Can you work these out from the model? Positions are in its coordinate system, mm. Coordinates: 2 decimals unless noted, no trailing zeros. Order: outer loops, then holes, each group sorted by start corner. A loop starts at its lowest first (then second) coordinate and runs counter-clockwise, first axis right, second up.
```python
from build123d import *

# Parameters (mm, degrees)
SKETCH1_W           = 65
SKETCH1_H           = 75
SKETCH1_R           = 2.75
SKETCH1_R_2         = 6
BOSS_EXTRUDE1_DEPTH = 5
CHAMFER1_SIZE       = 3
CUT_EXTRUDE1_REACH  = 58.789
SKETCH2_R           = 2.75
CUT_EXTRUDE2_REACH  = 58.789
SKETCH3_W           = 28
SKETCH3_H           = 20
FILLET1_R           = 40


with BuildPart() as part:
    # Sketch1 → Boss-Extrude1 (new body)
    with BuildSketch(Plane(origin=(600.828774839, 0, 0), x_dir=(0, -1, 0), z_dir=(-1, 0, 0))):
        with Locations((7.5, -2.5)):
            Rectangle(SKETCH1_W, SKETCH1_H)
        with Locations((30, -5)):
            Circle(SKETCH1_R, mode=Mode.SUBTRACT)
        with Locations(Location((-10, 25, 0), (0, 0, 180))):
            Circle(SKETCH1_R, mode=Mode.SUBTRACT)
        with Locations(Location((30, -25, 0), (0, 0, 180))):
            Circle(SKETCH1_R, mode=Mode.SUBTRACT)
        with Locations(Location((0, -10, 0), (0, 0, 180))):
            Circle(SKETCH1_R_2, mode=Mode.SUBTRACT)
    extrude(amount=-BOSS_EXTRUDE1_DEPTH)

    # Chamfer1
    chamfer1_edges = [part.edges().sort_by_distance(p)[0] for p in [
        (603.328774839, 25, 35),
        (603.328774839, -40, 35),
        (603.328774839, -40, -40),
    ]]
    chamfer(chamfer1_edges, length=CHAMFER1_SIZE)

    # Sketch2 → Cut-Extrude1 (cut, up to next)
    with BuildSketch(Plane.ZY.offset(-600.828774839), mode=Mode.PRIVATE) as cut_extrude1_sk1:
        with Locations(Location((4.405677967, 11.204416197, 0), (0, 0, 270))):
            Circle(SKETCH2_R)
    cut_extrude1_tool1 = extrude(cut_extrude1_sk1.sketch, amount=-CUT_EXTRUDE1_REACH, mode=Mode.PRIVATE) & part.part
    # Sketch2 → Cut-Extrude1 (cut, up to next)
    with BuildSketch(Plane.ZY.offset(-600.828774839), mode=Mode.PRIVATE) as cut_extrude1_sk2:
        with Locations(Location((-24.405677967, -11.204416197, 0), (0, 0, 270))):
            Circle(SKETCH2_R)
    cut_extrude1_tool2 = extrude(cut_extrude1_sk2.sketch, amount=-CUT_EXTRUDE1_REACH, mode=Mode.PRIVATE) & part.part
    add(cut_extrude1_tool1.solids().sort_by_distance((600.828775, 11.204416, 4.405678))[0], mode=Mode.SUBTRACT)
    add(cut_extrude1_tool2.solids().sort_by_distance((600.828775, -11.204416, -24.405678))[0], mode=Mode.SUBTRACT)

    # Sketch3 → Cut-Extrude2 (cut, up to next)
    with BuildSketch(Plane.ZY.offset(-600.828774839), mode=Mode.PRIVATE) as cut_extrude2_sk1:
        with Locations((21, -30)):
            Rectangle(SKETCH3_W, SKETCH3_H)
    cut_extrude2_tool1 = extrude(cut_extrude2_sk1.sketch, amount=-CUT_EXTRUDE2_REACH, mode=Mode.PRIVATE) & part.part
    add(cut_extrude2_tool1.solids().sort_by_distance((600.828775, -30, 21))[0], mode=Mode.SUBTRACT)

    # Fillet1
    fillet1_edges = [part.edges().sort_by_distance(p)[0] for p in [
        (603.328774839, 25, -40),
    ]]
    fillet(fillet1_edges, radius=FILLET1_R)


solid = part.part
```
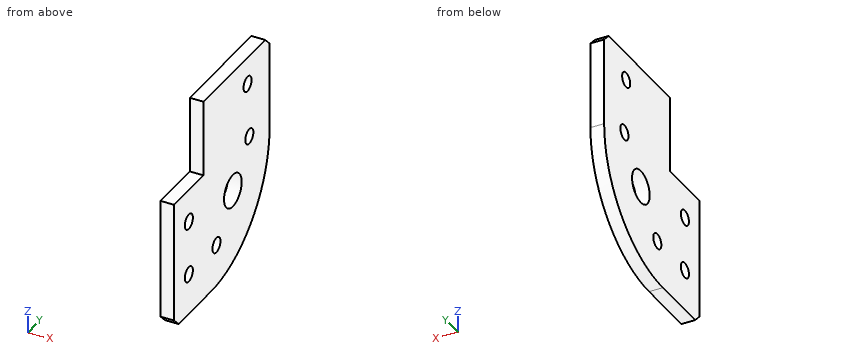
1. Please list where these lines run through material, in increasing order: probe 1 along Z at (x, y) = (602, -30); probe 2 along Z at (x, y) = (603.25, -28); probe 3 along Y at (x, z) = (601.5, -6).
Completed:
probe 1: z = -40 to -27.75, -22.25 to -7.75, -2.25 to 7
probe 2: z = -40 to -26.89, -23.11 to -6.89, -3.11 to 7
probe 3: y = -40 to -32.56, -27.44 to -4.47, 4.47 to 24.55
2. Imagine slicing it at A-A on y = -30. Please give me the cut outline in (x, z), then the cut area to 3 significant figures.
Completed:
outline: (600.83, -40) - (605.83, -40) - (605.83, -27.75) - (600.83, -27.75) - close; (600.83, -22.25) - (605.83, -22.25) - (605.83, -7.75) - (600.83, -7.75) - close; (600.83, -2.25) - (605.83, -2.25) - (605.83, 7) - (600.83, 7) - close
area: 180 mm2
3. Imagine slicing it at C-C on z = -5. Please give me the cut outline in (x, y).
Completed:
outline: (600.83, -40) - (605.83, -40) - (605.83, -32.75) - (600.83, -32.75) - close; (600.83, -27.25) - (605.83, -27.25) - (605.83, -3.32) - (600.83, -3.32) - close; (600.83, 3.32) - (605.83, 3.32) - (605.83, 24.69) - (600.83, 24.69) - close
4. I'm going to push flat-ended pins straight in: pin 1 (1 mm diameter, centred on x = 602.5, y = 4, fed in from -Z); pin 2 (1.5 mm diameter, centred on x = 603.5, z = -1.5, fed in from +Y); pin 3 (2.5 mm diameter, centred on x = 603, z = 23.5, fed in from -Y). Where does each tip first touch, or does it pass through?
Completed:
pin 1: stops at z = -35.46
pin 2: stops at y = 24.99
pin 3: stops at y = -20
5. Imagine slicing it at B-B on x = 602.8. Please give me the cut outline in (y, z), then the cut area to 3 significant figures.
Completed:
outline: (-40, -37) - (-37, -40) - (-15, -40) arc R40 ccw to (25, 0) - (25, 32) - (22, 35) - (-20, 35) - (-20, 7) - (-40, 7) - close; hole circle Ø5.5 at (-30, -25); hole circle Ø5.5 at (-30, -5); hole circle Ø5.5 at (-11.2, -24.41); hole circle Ø12 at (0, -10); hole circle Ø5.5 at (10, 25); hole circle Ø5.5 at (11.2, 4.41)
area: 3,730 mm2
6. Imagine slicing it at D-D on z = 20.5. Please give me the cut outline in (x, y).
Completed:
outline: (600.83, -20) - (605.83, -20) - (605.83, 25) - (600.83, 25) - close
